The listing builds one solid part. Answer for the finished solid, in the listing's coordinates (mm). Round coordinates to 2 decimals unless told otherwise and drop trailing zeros. Write each loop counter-clockwise with the first axis right and the second up, starting at its lowest first coordinate (ties: lowest second). Pieces come first, ordered by that corner, then holes.
Item 1: Find section A-A on x = 61. Give the vertices of the cut face in (y, z), then the cut area to 3 significant figures.
Item 2: Find section D-D on y = -0.5. Give the vertices of the cut face in (x, z).
Item 3: Each of these flat-tipped pins is pushed along its axis until it touches: pin 1 (1.5 mm diameter, centred on y = 7, z = 2, fed in from -X); pin 2 (10 mm diameter, centred on x = -31.5, y = 6.5, fed in from -Z); pin 3 (2 mm diameter, centred on x = -3.5, z = 2, fed in from +Y); pin 4 (1 mm diameter, centred on x = 37, z = 3, fed in from -Y). Where does it stop, or does it pass through?
Item 4: Find section B-B on y = -10. Give the vertices of the cut face in (x, z).
Item 5: Find the intervals of material crossed by probe 1 along X at (y, z) = (0, 4.85); probe 2 along Y at (x, z) = (-47, 2.65); probe 3 along X at (y, z) = (1, 1.1), in increasing order.
Item 6: Find section C-C on z = 4.55. Give the vertices of the cut face in (x, y), then the cut area to 3 significant figures.
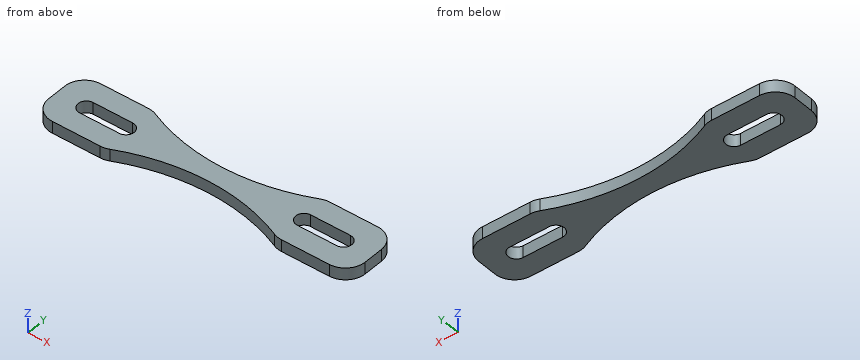
```python
from build123d import *

# Parameters (mm, degrees)
BOSS_EXTRUDE1_DEPTH = 6
FILLET1_R           = 10


with BuildPart() as part:
    # Sketch1 → Boss-Extrude1 (new body)
    with BuildSketch(Plane.XY):
        with BuildLine():
            Line((-80, -15), (-43.588989435, -15))
            ThreePointArc((-43.588989435, -15), (0, -5), (43.588989435, -15))
            Line((43.588989435, -15), (80, -15))
            Line((80, -15), (80, 15))
            Line((80, 15), (43.588989435, 15))
            ThreePointArc((43.588989435, 15), (0, 5), (-43.588989435, 15))
            Line((-43.588989435, 15), (-80, 15))
            Line((-80, 15), (-80, -15))
        make_face()
        with BuildLine():
            Line((-65, 4.15), (-45, 4.15))
            ThreePointArc((-45, 4.15), (-40.85, 0), (-45, -4.15))
            Line((-45, -4.15), (-65, -4.15))
            ThreePointArc((-65, -4.15), (-69.15, 0), (-65, 4.15))
        make_face(mode=Mode.SUBTRACT)
        with BuildLine():
            Line((65, 4.15), (45, 4.15))
            ThreePointArc((45, 4.15), (40.85, 0), (45, -4.15))
            Line((45, -4.15), (65, -4.15))
            ThreePointArc((65, -4.15), (69.15, 0), (65, 4.15))
        make_face(mode=Mode.SUBTRACT)
    extrude(amount=BOSS_EXTRUDE1_DEPTH)

    # Fillet1
    fillet1_edges = [part.edges().sort_by_distance(p)[0] for p in [
        (80, 15, 3),
        (80, -15, 3),
        (43.588989435, -15, 3),
        (-43.588989435, -15, 3),
        (-80, -15, 3),
        (-80, 15, 3),
        (-43.588989435, 15, 3),
        (43.588989435, 15, 3),
    ]]
    fillet(fillet1_edges, radius=FILLET1_R)


solid = part.part
```
Check values:
1. outline: (-15, 0) - (-4.15, 0) - (-4.15, 6) - (-15, 6) - close; (4.15, 0) - (15, 0) - (15, 6) - (4.15, 6) - close
1. area: 130 mm2
2. outline: (-80, 0) - (-69.12, 0) - (-69.12, 6) - (-80, 6) - close; (-40.88, 0) - (40.88, 0) - (40.88, 6) - (-40.88, 6) - close; (69.12, 0) - (80, 0) - (80, 6) - (69.12, 6) - close
3. pin 1: stops at x = -79.92
3. pin 2: stops at z = 0
3. pin 3: stops at y = 5.1
3. pin 4: stops at y = -12.3
4. outline: (-78.66, 0) - (-31.22, 0) - (-31.22, 6) - (-78.66, 6) - close; (31.22, 0) - (78.66, 0) - (78.66, 6) - (31.22, 6) - close
5. probe 1: x = -80 to -69.15, -40.85 to 40.85, 69.15 to 80
5. probe 2: y = -15 to -4.15, 4.15 to 15
5. probe 3: x = -80 to -69.03, -40.97 to 40.97, 69.03 to 80
6. outline: (-80, -5) arc R10 ccw to (-70, -15) - (-45.83, -15) arc R10 ccw to (-41.66, -14.09) arc R100 cw to (41.66, -14.09) arc R10 ccw to (45.83, -15) - (70, -15) arc R10 ccw to (80, -5) - (80, 5) arc R10 ccw to (70, 15) - (45.83, 15) arc R10 ccw to (41.66, 14.09) arc R100 cw to (-41.66, 14.09) arc R10 ccw to (-45.83, 15) - (-70, 15) arc R10 ccw to (-80, 5) - close; hole (-65, -4.15) - (-45, -4.15) arc R4.15 ccw to (-45, 4.15) - (-65, 4.15) arc R4.15 ccw to start; hole (45, -4.15) - (65, -4.15) arc R4.15 ccw to (65, 4.15) - (45, 4.15) arc R4.15 ccw to start
6. area: 3,100 mm2
